from build123d import *

# Parameters (mm, degrees)
SKETCH_W        = 100
SKETCH_H        = 100
PAD_DEPTH       = 5
SKETCH001_R     = 4.5
POCKET_DEPTH    = 2
SKETCH002_R     = 2.5
POCKET001_DEPTH = 3
SKETCH003_R     = 2.625
POCKET002_DEPTH = 5
FILLET_R        = 10


with BuildPart() as part:
    # Sketch → Pad (new body)
    with BuildSketch(Plane.XY):
        Rectangle(SKETCH_W, SKETCH_H)
    extrude(amount=PAD_DEPTH)

    # Sketch001 (on Face6 of Pad) → Pocket (cut)
    with BuildSketch(Plane.XY.offset(5)):
        with Locations((0, 10)):
            Circle(SKETCH001_R)
        with Locations((10, 0)):
            Circle(SKETCH001_R)
        with Locations((-10, 0)):
            Circle(SKETCH001_R)
        with Locations((0, -10)):
            Circle(SKETCH001_R)
    extrude(amount=-POCKET_DEPTH, mode=Mode.SUBTRACT)

    # Sketch002 (on Face4 of Pocket) → Pocket001 (cut)
    with BuildSketch(Plane(origin=(0, 0, 0), x_dir=(1, 0, 0), z_dir=(0, 0, -1))):
        with Locations((0, 10)):
            Circle(SKETCH002_R)
        with Locations((10, 0)):
            Circle(SKETCH002_R)
        with Locations((0, -10)):
            Circle(SKETCH002_R)
        with Locations((-10, 0)):
            Circle(SKETCH002_R)
    extrude(amount=-POCKET001_DEPTH, mode=Mode.SUBTRACT)

    # Sketch003 (on Face5 of Pocket001) → Pocket002 (cut)
    with BuildSketch(Plane.XY.offset(5)):
        with Locations((-40, 0)):
            Circle(SKETCH003_R)
        with Locations((-40, -40)):
            Circle(SKETCH003_R)
        with Locations((-40, -20)):
            Circle(SKETCH003_R)
        with Locations((-20, -40)):
            Circle(SKETCH003_R)
        with Locations((0, -40)):
            Circle(SKETCH003_R)
        with Locations((20, -40)):
            Circle(SKETCH003_R)
        with Locations((40, -40)):
            Circle(SKETCH003_R)
        with Locations((40, -20)):
            Circle(SKETCH003_R)
        with Locations((40, 0)):
            Circle(SKETCH003_R)
        with Locations((40, 20)):
            Circle(SKETCH003_R)
        with Locations((40, 40)):
            Circle(SKETCH003_R)
        with Locations((20, 40)):
            Circle(SKETCH003_R)
        with Locations((0, 40)):
            Circle(SKETCH003_R)
        with Locations((-20, 40)):
            Circle(SKETCH003_R)
        with Locations((-40, 40)):
            Circle(SKETCH003_R)
        with Locations((-40, 20)):
            Circle(SKETCH003_R)
    extrude(amount=-POCKET002_DEPTH, mode=Mode.SUBTRACT)

    # Fillet
    fillet_edges = [part.edges().sort_by_distance(p)[0] for p in [
        (-50, 50, 2.5),
        (50, 50, 2.5),
        (50, -50, 2.5),
        (-50, -50, 2.5),
    ]]
    fillet(fillet_edges, radius=FILLET_R)


solid = part.part
Check sheet for the modelled part. Datum: model origin and axes. Units: mm. A direction names the side the tool comes from. Give positions to 0.01 mm unless a question says otherwise; leave off trailing zeros. Write each loop counter-clockwise with the first axis right and the second up, starting at its lowest first coordinate (ties: lowest second). Pieces come first, ordered by that corner, then holes. Notation, with made-up numbers: (49.5, -24) -> (96.5, -24) arc R32 ccw to (96.5, 14) -> close; hole circle Ø1 at (10.5, 41). An arc over 180 degrees is marked (long way). Write item = value, one per line.
Item 1: Scan lines: probe 1 along Y at (x, z) = (20, 1.4) (3 decimals); probe 2 along X at (y, z) = (2, 2.35); probe 3 along Y at (x, z) = (12, 0.75). Record each from-to range of solid material in increasing order. Write a range as from..to.
Output:
probe_1 = -50..-42.625, -37.375..37.375, 42.625..50
probe_2 = -50..-41.7, -38.3..-11.5, -8.5..8.5, 11.5..38.3, 41.7..50
probe_3 = -50..-1.5, 1.5..50
Item 2: Release check for a two-part mould opening along Y. For faces 3 (the flat face through (-1, 50, 2)), 4 (the cylindrical face through (-47.15, -46.99, 2.54)), 5 (the cylindrical face through (17.92, 38.4, 2.54)), 6 (the flat face through (50, -1, 2)) record: +Y half, -Y half, draft (parallel to the pull), parting line (faces both ways), or undercut.
Output:
face_3 = +Y half
face_4 = -Y half
face_5 = undercut
face_6 = draft
Item 3: Sectioned sample at A-A on y = -10. Record the boundary of the cut face in (x, z), and give its area (3 significant figures).
Output:
outline = (-50, 0) -> (-2.5, 0) -> (-2.5, 3) -> (-4.5, 3) -> (-4.5, 5) -> (-50, 5) -> close; (2.5, 0) -> (50, 0) -> (50, 5) -> (4.5, 5) -> (4.5, 3) -> (2.5, 3) -> close
area = 467 mm^2
Item 4: Tool access check on faces 1 (the cylindrical face through (-22.08, 38.4, 2.54)), 2 (the cylindrical face through (-5.708, 1.352, 4.014)). Record the directions out of +Z, -Z, +X, -X, +Y, -Y that give a thin tool (end or side, any length) a straight path to the whole face; none if there is none.
Output:
face_1 = +Z, -Z
face_2 = +Z
Item 5: Sectioned sample at C-C on x = 20. Record the boundary of the cut face in (y, z) (3 decimals), and give its area (4 significant figures).
Output:
outline = (-50, 0) -> (-42.625, 0) -> (-42.625, 5) -> (-50, 5) -> close; (-37.375, 0) -> (37.375, 0) -> (37.375, 5) -> (-37.375, 5) -> close; (42.625, 0) -> (50, 0) -> (50, 5) -> (42.625, 5) -> close
area = 447.5 mm^2
Item 6: Gauge pin test, flat end, axial feed: pin 1 (4.5 mm diameter, centred on x = 1.5, y = 8.5, fed in from +Z). Record the tip position at first contact, or that the pin passes through.
Output:
pin_1 = 3
